The listing builds one solid part. Answer for the finished solid, in the listing's coordinates (mm). A direction names the side the tool comes from. Coordinates: 2 decimals unless noted, no trailing zeros. Loops run counter-clockwise (first coordinate to the right, second up) from the corner with the lowest first, then second, coordinate; pieces in that order, holes last. Notation, with made-up numbers: M 12,0 L 31,0 A34 ccw 31,33 Z; hole C 24.25,-37 d8. An arc over 180 degrees is marked long. Answer as a JSON object with one key per item and string values. Group by question number.
1. A cutting plane is placed at C-C on y = 25. Give the vertices of the cut face in (x, z).
2. A cutting plane is placed at A-A on z = 56.5. Give the vertices of the cut face in (x, y).
3. For faces 4 (the face through (55.333, 62.825, -90.507)), 5 (the face through (25, 135, -55)), 6 (the face through (0, 138, 0)), determine the directions among +Z, -Z, +X, -X, +Y, -Y from which every point of the face is accessible in a straight line to the end or side of a thin tool.
4. Given pin 1 (1 mm diameter, centred on x = 17, z = -40, fed in from -Y); pin 2 (10 mm diameter, centred on y = 71.5, z = -43, fed in from +X); pin 3 (3 mm diameter, centred on x = 31, y = 110, fed in from +Z), each flat-ended and moving along its own axis, determine where each tip first touches the part or whether it passes through.
5. A cutting plane is placed at D-D on y = 170. Give the vertices of the cut face in (x, z), and give its area (3 significant figures).
6. A cutting plane is placed at B-B on x = 90. Give the vertices of the cut face in (y, z).
7. Straight lines are drawn through the part: L1, parallel to Y at x = -3, z = 56; L2, parallel to Z at x = -3.8, y = 25; L3, parallel to Z at x = -2.5, y = 250. For each, find the intervals that lie inside material, in ascending order.
8. Determine the mould class of faces 1 (the face through (-2.46, 26.96, -65.27)), 2 (the face through (25, 145, -55)), 3 (the face through (44, 138, -92.5)) for opening direction Z: released by +Z, released by -Z, zero draft, split by the parting line, or undercut.
from build123d import *

# Parameters (mm, degrees)
F1_DEPTH  = 280
F2_R      = 2
F3_R      = 4.25
F4_DEPTH  = 5.001
F5_W      = 10
F5_H      = 85
F6_DEPTH  = 65
F8_DEPTH  = 145.001
F9_R      = 10.25
F10_DEPTH = 5.001
F11_R     = 5
F12_R     = 2


# Not quite as in the source:
# - a feature names something its author has since deleted; it is built from what else it names


with BuildPart() as f1:
    # F0 (on Front) → F1 (new body)
    with BuildSketch(Plane.XZ):
        Polygon((0, 87.5), (-5, 87.5), (-5, -92.5), (115, -92.5), (115, -87.5), (0, -87.5), align=None)
    extrude(amount=-F1_DEPTH)

    # F2
    f2_edges = [f1.edges().sort_by_distance(p)[0] for p in [
        (-2.5, 280, 87.5),
        (-2.5, 0, 87.5),
    ]]
    fillet(f2_edges, radius=F2_R)

    # F3 (on face) → F4 (cut, through all)
    with BuildSketch(Plane.YZ):
        with Locations((25, 56.5)):
            Circle(F3_R)
        with Locations((25, -61.5)):
            Circle(F3_R)
        with Locations((250, -61.5)):
            Circle(F3_R)
        with Locations((250, 56.5)):
            Circle(F3_R)
    extrude(amount=-F4_DEPTH, mode=Mode.SUBTRACT)

    # F5 (on face) → F6 (join)
    with BuildSketch(Plane.YZ):
        with Locations((140, -45)):
            Rectangle(F5_W, F5_H)
    extrude(amount=F6_DEPTH)

    # F7 (on face) → F8 (cut, through all)
    with BuildSketch(Plane(origin=(0, 145, 0), x_dir=(-1, 0, 0), z_dir=(0, 1, 0))):
        Polygon((-65, -87.5), (0, -2.5), (-65, -2.5), align=None)
    extrude(amount=-F8_DEPTH, mode=Mode.SUBTRACT)

    # F9 (on face) → F10 (cut, through all)
    with BuildSketch(Plane.XY.offset(-87.5)):
        with Locations((90, 140)):
            Circle(F9_R)
        with BuildLine():
            ThreePointArc((109.1388440622, 156.0842981806), (113.4890517215, 148.5594654753), (115, 140))
            Line((115, 140), (115, 280))
            Line((115, 280), (0, 280))
            Line((0, 280), (109.1388440622, 156.0842981806))
        make_face()
        with BuildLine():
            ThreePointArc((115, 140), (113.4890517215, 131.4405345247), (109.1388440622, 123.9157018194))
            Line((109.1388440622, 123.9157018194), (0, 0))
            Line((0, 0), (115, 0))
            Line((115, 0), (115, 140))
        make_face()
    extrude(amount=-F10_DEPTH, mode=Mode.SUBTRACT)

    # F11
    f11_edges = [f1.edges().sort_by_distance(p)[0] for p in [
        (-5, 140, -92.5),
    ]]
    fillet(f11_edges, radius=F11_R)

    # F12
    f12_edges = [f1.edges().sort_by_distance(p)[0] for p in [
        (0, 212.5, -87.5),
        (0, 67.5, -87.5),
    ]]
    fillet(f12_edges, radius=F12_R)


solid = f1.part
From the geometry:
{
 "1": {"outline": "M -5,-87.5 A5 ccw 0,-92.5 L 22.02,-92.5 L 22.02,-87.5 L 2,-87.5 A2 cw 0,-85.5 L 0,-65.75 L -5,-65.75 Z; M -5,-57.25 L 0,-57.25 L 0,52.25 L -5,52.25 Z; M -5,60.75 L 0,60.75 L 0,87.5 L -5,87.5 Z"},
 "2": {"outline": "M -5,0 L 0,0 L 0,20.75 L -5,20.75 Z; M -5,29.25 L 0,29.25 L 0,245.75 L -5,245.75 Z; M -5,254.25 L 0,254.25 L 0,280 L -5,280 Z"},
 "3": {"face 4": "+Z, -Z, +X, -Y", "face 5": "+Z, +X, -Y", "face 6": "+Z, +X"},
 "4": {"pin 1": "stops at y = 135", "pin 2": "stops at x = 0", "pin 3": "stops at z = -87.5"},
 "5": {"outline": "M -5,-87.5 A5 ccw 0,-92.5 L 96.88,-92.5 L 96.88,-87.5 L 2,-87.5 A2 cw 0,-85.5 L 0,87.5 L -5,87.5 Z", "area": "1,380 mm²"},
 "6": {"outline": "M 102.19,-92.5 L 129.75,-92.5 L 129.75,-87.5 L 102.19,-87.5 Z; M 150.25,-92.5 L 177.81,-92.5 L 177.81,-87.5 L 150.25,-87.5 Z"},
 "7": {"L1": "y = 0 to 20.78, 29.22 to 245.78, 254.22 to 280", "L2": "z = -90.75 to -65.75, -57.25 to 52.25, 60.75 to 87.5", "L3": "z = -91.83 to -65.75, -57.25 to 52.25, 60.75 to 87.5"},
 "8": {"face 1": "undercut", "face 2": "zero draft", "face 3": "released by -Z"}
}
